The model under review builds one solid part; all positions refer to its coordinate system, in mm. Coordinates: 2 decimals unless noted, no trailing zeros. Write each loop counter-clockwise with the first axis right and the second up, starting at its lowest first coordinate (ties: lowest second). Pieces come first, ordered by that corner, then holes. Notation, with made-up numbers: (9, -13) - (54, -13) arc R21 ccw to (54, -2) - close; hole circle Ø8 at (-9, -27.5). An arc over 180 degrees is marked (long way). Return JSON: item names as keys, results as strings. Group by question number.
(1) We need section C-C on x = -10. State the section outline as (y, z) points, then the cut area to 3 significant figures.
(2) We need section B-B on y = -2. State the section outline as (x, z) points.
(3) We need section D-D on x = -88. State the section outline as (y, z) points, then the cut area to 3 significant figures.
(4) For pin 1 Ø2.5 at (y, z) = (-1.5, 35) entering from +X, flat-tipped, find the tip position at first contact; note if it passes through.
(5) To check wall thickness, follow L1, parallel to X at y = 2.5, z = -2; L2, parallel to Z at x = -30, y = -0.25; L3, parallel to Z at x = 30, y = 0.5. State the ranges of each line that lie inside material, in increasing order. Write a range as from..to.
(6) We need section A-A on x = 30. State the section outline as (y, z) points, then the cut area to 3 significant figures.
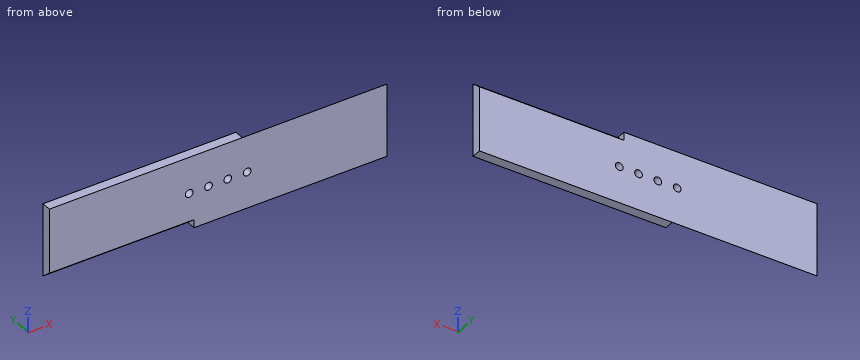
```python
from build123d import *

# Parameters (mm, degrees)
SKETCH1_W             = 350
SKETCH1_H             = 75
BOSS_EXTRUDE2_DEPTH   = 5
F_8_0MM_DOWEL_HOLE1_D = 8
CUT_EXTRUDE3_DEPTH    = 150
CUT_EXTRUDE4_DEPTH    = 150


with BuildPart() as part:
    # Sketch1 → Boss-Extrude2 (new, symmetric)
    with BuildSketch(Plane(origin=(0, 0, 0), x_dir=(1, 0, 0), z_dir=(0, 1, 0))):
        Rectangle(SKETCH1_W, SKETCH1_H)
    extrude(amount=BOSS_EXTRUDE2_DEPTH, both=True)

    # Ø8.0mm Dowel Hole1 (through all)
    with Locations(Plane(origin=(0, 5, 0), x_dir=(1, 0, 0), z_dir=(0, 1, 0))):
        with Locations((10, 0), (30, 0), (-10, 0), (-30, 0)):
            Hole(F_8_0MM_DOWEL_HOLE1_D / 2)

    # Sketch10 → Cut-Extrude3 (cut)
    with BuildSketch(Plane(origin=(175, 0, 0), x_dir=(0, 0, -1), z_dir=(1, 0, 0))):
        Polygon((-37.5, 5), (-37.5, -5), (-29.109003688, 5), align=None)
    extrude(amount=-CUT_EXTRUDE3_DEPTH, mode=Mode.SUBTRACT)

    # Sketch11 → Cut-Extrude4 (cut)
    with BuildSketch(Plane.ZY.offset(175)):
        Polygon((-37.5, 5), (-37.5, -5), (-29.109003688, -5), align=None)
    extrude(amount=-CUT_EXTRUDE4_DEPTH, mode=Mode.SUBTRACT)


solid = part.part
```
Ans:
{
 "1": {"outline": "(-5, -37.5) - (5, -37.5) - (5, -4) - (-5, -4) - close; (-5, 4) - (5, 4) - (5, 37.5) - (-5, 37.5) - close", "area": "670 mm²"},
 "2": {"outline": "(-175, -31.63) - (-25, -31.63) - (-25, -37.5) - (175, -37.5) - (175, 34.98) - (25, 34.98) - (25, 37.5) - (-175, 37.5) - close; hole circle Ø8 at (-30, 0); hole circle Ø8 at (-10, 0); hole circle Ø8 at (10, 0); hole circle Ø8 at (30, 0)"},
 "3": {"outline": "(-5, -29.11) - (5, -37.5) - (5, 37.5) - (-5, 37.5) - close", "area": "708 mm²"},
 "4": {"pin 1": "x = 175"},
 "5": {"L1": "-175..-33.46, -26.54..-13.46, -6.54..6.54, 13.46..26.54, 33.46..175", "L2": "-33.09..-4, 4..37.5", "L3": "-37.5..-4, 4..32.88"},
 "6": {"outline": "(-5, -37.5) - (5, -37.5) - (5, -4) - (-5, -4) - close; (-5, 4) - (5, 4) - (5, 29.11) - (-5, 37.5) - close", "area": "628 mm²"}
}
